Model file for the job. Use its own axes, mm. Round coordinates to 2 decimals unless told otherwise and drop trailing zeros. Loops run counter-clockwise (first coordinate to the right, second up) from the corner with the lowest first, then second, coordinate; pieces in that order, holes last. Notation, with made-up numbers: (19, 31) - (78, 31) arc R18 ccw to (78, 44) - close; hole circle Ø7 at (-30, 83). An arc over 180 degrees is marked (long way). Answer as a JSON object with one key per item and string values.
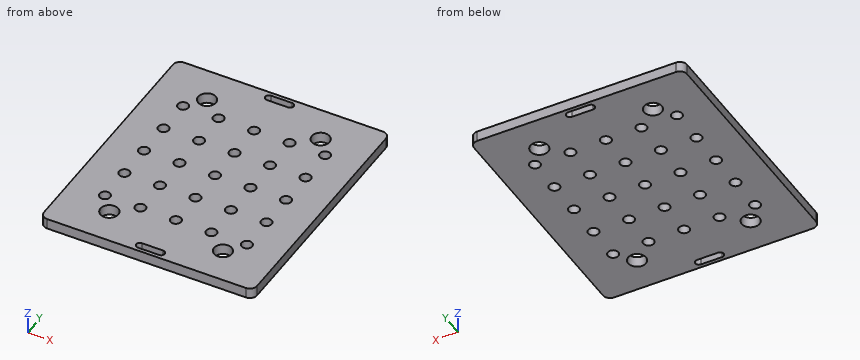
from build123d import *

# Parameters (mm, degrees)
MODEL_R             = 1.5
MODEL_R_2           = 2.5
BOSS_EXTRUDE1_DEPTH = 3


with BuildPart() as part:
    # Model → Boss-Extrude1 (new body)
    with BuildSketch(Plane.XY):
        with BuildLine():
            Line((-2, 70), (-58, 70))
            ThreePointArc((-58, 70), (-59.414213562, 69.414213562), (-60, 68))
            Line((-60, 68), (-60, 2))
            ThreePointArc((-60, 2), (-59.414213562, 0.585786438), (-58, 0))
            Line((-58, 0), (-2, 0))
            ThreePointArc((-2, 0), (-0.585786438, 0.585786438), (0, 2))
            Line((0, 2), (0, 68))
            ThreePointArc((0, 68), (-0.585786438, 69.414213562), (-2, 70))
        make_face()
        with Locations((-20, 45)):
            Circle(MODEL_R, mode=Mode.SUBTRACT)
        with Locations((-10, 35)):
            Circle(MODEL_R, mode=Mode.SUBTRACT)
        with Locations((-50, 45)):
            Circle(MODEL_R, mode=Mode.SUBTRACT)
        with Locations((-20, 15)):
            Circle(MODEL_R, mode=Mode.SUBTRACT)
        with Locations((-20, 35)):
            Circle(MODEL_R, mode=Mode.SUBTRACT)
        with Locations((-40, 25)):
            Circle(MODEL_R, mode=Mode.SUBTRACT)
        with Locations((-40, 15)):
            Circle(MODEL_R, mode=Mode.SUBTRACT)
        with Locations((-30, 25)):
            Circle(MODEL_R, mode=Mode.SUBTRACT)
        with Locations((-40, 55)):
            Circle(MODEL_R, mode=Mode.SUBTRACT)
        with Locations((-10, 25)):
            Circle(MODEL_R, mode=Mode.SUBTRACT)
        with Locations((-30, 45)):
            Circle(MODEL_R, mode=Mode.SUBTRACT)
        with Locations((-10, 55)):
            Circle(MODEL_R, mode=Mode.SUBTRACT)
        with Locations((-10, 45)):
            Circle(MODEL_R, mode=Mode.SUBTRACT)
        with Locations((-50, 15)):
            Circle(MODEL_R, mode=Mode.SUBTRACT)
        with Locations((-10, 15)):
            Circle(MODEL_R, mode=Mode.SUBTRACT)
        with Locations((-50, 35)):
            Circle(MODEL_R, mode=Mode.SUBTRACT)
        with Locations((-40, 45)):
            Circle(MODEL_R, mode=Mode.SUBTRACT)
        with Locations((-30, 15)):
            Circle(MODEL_R, mode=Mode.SUBTRACT)
        with Locations((-30, 35)):
            Circle(MODEL_R, mode=Mode.SUBTRACT)
        with Locations((-40, 35)):
            Circle(MODEL_R, mode=Mode.SUBTRACT)
        with Locations((-20, 25)):
            Circle(MODEL_R, mode=Mode.SUBTRACT)
        with Locations((-50, 25)):
            Circle(MODEL_R, mode=Mode.SUBTRACT)
        with Locations((-50, 55)):
            Circle(MODEL_R, mode=Mode.SUBTRACT)
        with Locations((-30, 55)):
            Circle(MODEL_R, mode=Mode.SUBTRACT)
        with Locations((-20, 55)):
            Circle(MODEL_R, mode=Mode.SUBTRACT)
        with Locations((-46, 60)):
            Circle(MODEL_R_2, mode=Mode.SUBTRACT)
        with Locations((-14, 10)):
            Circle(MODEL_R_2, mode=Mode.SUBTRACT)
        with Locations((-14, 60)):
            Circle(MODEL_R_2, mode=Mode.SUBTRACT)
        with Locations((-46, 10)):
            Circle(MODEL_R_2, mode=Mode.SUBTRACT)
        with BuildLine():
            Line((-27, 1), (-33, 1))
            ThreePointArc((-33, 1), (-34, 2), (-33, 3))
            Line((-33, 3), (-27, 3))
            ThreePointArc((-27, 3), (-26, 2), (-27, 1))
        make_face(mode=Mode.SUBTRACT)
        with BuildLine():
            Line((-33, 68.999828109), (-27, 68.999828109))
            ThreePointArc((-27, 68.999828109), (-26, 67.999828109), (-27, 66.999828109))
            Line((-27, 66.999828109), (-33, 66.999828109))
            ThreePointArc((-33, 66.999828109), (-34, 67.999828109), (-33, 68.999828109))
        make_face(mode=Mode.SUBTRACT)
    extrude(amount=BOSS_EXTRUDE1_DEPTH)


solid = part.part
1) Slice it at D-D on y = 45. List the corners of the cut face in (x, z).
Values follow:
{"outline": "(-60, 0) - (-51.5, 0) - (-51.5, 3) - (-60, 3) - close; (-48.5, 0) - (-41.5, 0) - (-41.5, 3) - (-48.5, 3) - close; (-38.5, 0) - (-31.5, 0) - (-31.5, 3) - (-38.5, 3) - close; (-28.5, 0) - (-21.5, 0) - (-21.5, 3) - (-28.5, 3) - close; (-18.5, 0) - (-11.5, 0) - (-11.5, 3) - (-18.5, 3) - close; (-8.5, 0) - (0, 0) - (0, 3) - (-8.5, 3) - close"}
2) Slice it at C-C on x = -14. List the corners of the cut face in (y, z), then the cut area to 3 significant figures.
Values follow:
{"outline": "(0, 0) - (7.5, 0) - (7.5, 3) - (0, 3) - close; (12.5, 0) - (57.5, 0) - (57.5, 3) - (12.5, 3) - close; (62.5, 0) - (70, 0) - (70, 3) - (62.5, 3) - close", "area": "180 mm²"}
3) Slice it at A-A on x = -40. List the corners of the cut face in (y, z), then the cut area to 3 significant figures.
Values follow:
{"outline": "(0, 0) - (13.5, 0) - (13.5, 3) - (0, 3) - close; (16.5, 0) - (23.5, 0) - (23.5, 3) - (16.5, 3) - close; (26.5, 0) - (33.5, 0) - (33.5, 3) - (26.5, 3) - close; (36.5, 0) - (43.5, 0) - (43.5, 3) - (36.5, 3) - close; (46.5, 0) - (53.5, 0) - (53.5, 3) - (46.5, 3) - close; (56.5, 0) - (70, 0) - (70, 3) - (56.5, 3) - close", "area": "165 mm²"}
4) Slice it at B-B on y = 58.5. List the corners of the cut face in (x, z), then the cut area to 3 significant figures.
Values follow:
{"outline": "(-60, 0) - (-48, 0) - (-48, 3) - (-60, 3) - close; (-44, 0) - (-16, 0) - (-16, 3) - (-44, 3) - close; (-12, 0) - (0, 0) - (0, 3) - (-12, 3) - close", "area": "156 mm²"}
5) Probe probe 1 along Y at (x, z) = (-20, 0.8); probe 2 along Y at (x, z) = (-32, 2.8); probe 3 along X at (y, z) = (54, 1.75). List the from-to ranges inside material, lowest first.
Values follow:
{"probe 1": "0 to 13.5, 16.5 to 23.5, 26.5 to 33.5, 36.5 to 43.5, 46.5 to 53.5, 56.5 to 70", "probe 2": "0 to 1, 3 to 67, 69 to 70", "probe 3": "-60 to -51.12, -48.88 to -41.12, -38.88 to -31.12, -28.88 to -21.12, -18.88 to -11.12, -8.88 to 0"}
